Can you work these out from the model? Positions are in its coordinate system, mm. Face numbers are marked on the shaded views. A direction names the side the tool comes from. Round coordinates to 2 decimals unless told otherwise and drop trailing zeros. Order: outer loops, then holes, each group sorted by start corner. A loop starts at its lowest first (then second) coordinate and runs counter-clockwise, first axis right, second up. Notation, with made-up numbers: (53, 86) -> (89, 86) arc R17 cw to (89, 112) -> close; hole circle Ø11 at (-22, -2). An arc over 180 degrees is marked (long way). Use a Markdown table: item, result. Add a question column.
Q1. For the marked faces 1 and 2, which set-ups out of +Z, -Z, +X, -X, +Y, -Y let a thin tool reach every point of the face, with its end or its side?
Q2. I need wall thicknesses on line 1 along Y through (x, z) = (24.5, 23.5); line 2 along X through (y, z) = (32, 51.5). Which ranges of each line are inside material? Lowest first, please. Write a range as [from, to].
Q3. If we section it at A-A on x = 32.5: List the corners of the cut face in (y, z) for me, plus the area to 3 significant figures.
Q4. If we section it at C-C on x = 18: List the corners of the cut face in (y, z) for me.
Q5. If we section it at D-D on y = 38.1: List the corners of the cut face in (x, z) for me, plus the area to 3 significant figures.
Q6. I'm going to push flat-ended pins straight in: pin 1 Ø8 at (x, z) = (45.28, 47.62) entering from -Y; pin 2 Ø4 at (x, z) = (45.28, 47.62) entering from +Y; pin 3 Ø12 at (x, y) = (30, 64.5) entering from -Z. Where does each tip first touch, or does it pass through?
Q7. We'd pull the mould along Y, two halves only. Please class the marked faces 3, 4 and 5: +Y half, -Y half, draft (parallel to the pull), parting line (faces both ways), or undercut.
Q8. If we section it at B-B on z = 31: List the corners of the cut face in (x, y) for me, plus the area to 3 significant figures.
```python
from build123d import *

# Parameters (mm, degrees)
SKETCH2_W               = 50.8
SKETCH2_H               = 76.2
BOSS_EXTRUDE2_DEPTH     = 57.15
SKETCH3_R               = 38.1
CUT_EXTRUDE1_DEPTH      = 108.95
SHELL1_T                = -6.35
F_1_4_CLEARANCE_HOLE1_D = 6.7564


with BuildPart() as part:
    # Sketch2 → Boss-Extrude2 (new body)
    with BuildSketch(Plane.XY):
        with Locations((25.4, 38.1)):
            Rectangle(SKETCH2_W, SKETCH2_H)
    extrude(amount=BOSS_EXTRUDE2_DEPTH)

    # Sketch3 → Cut-Extrude1 (cut, through all)
    with BuildSketch(Plane(origin=(50.8, 0, 0), x_dir=(0, 0, -1), z_dir=(1, 0, 0))):
        with Locations((0, 38.1)):
            Circle(SKETCH3_R)
    extrude(amount=-CUT_EXTRUDE1_DEPTH, mode=Mode.SUBTRACT)

    # Shell1
    shell1_openings = [part.faces().sort_by_distance(p)[0] for p in [
        (25.4, 38.1, 57.15),
        (25.4, 38.1, 38.1),
        (50.8, 38.1, 42.20881959),
    ]]
    offset(amount=SHELL1_T, openings=shell1_openings, kind=Kind.INTERSECTION)

    # 1/4 Clearance Hole1 (through all)
    with Locations(Plane(origin=(0, 76.2, 0), x_dir=(1, 0, 0), z_dir=(0, 1, 0))):
        with Locations((45.28185, -47.625), (19.88185, -47.625)):
            Hole(F_1_4_CLEARANCE_HOLE1_D / 2)


solid = part.part
```
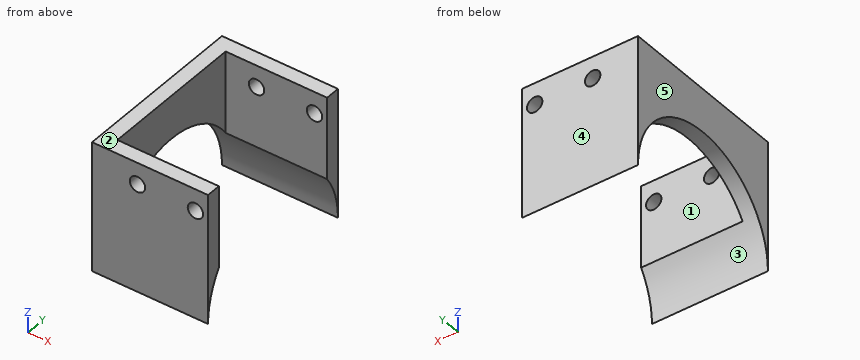
Answer below:
| question | item | result |
|---|---|---|
| 1 | face 1 | +Z, -Z, +X |
| 1 | face 2 | +Z, +X, -X, +Y, -Y |
| 2 | line 1 | [0, 6.35], [69.85, 76.2] |
| 2 | line 2 | [0, 6.35] |
| 3 | outline | (0, 0) arc R38.1 cw to (6.35, 21.06) -> (6.35, 57.15) -> (0, 57.15) -> close; (69.85, 21.06) arc R38.1 cw to (76.2, 0) -> (76.2, 57.15) -> (69.85, 57.15) -> close |
| 3 | area | 544 mm² |
| 4 | outline | (0, 0) arc R38.1 cw to (6.35, 21.06) -> (6.35, 44.82) -> (0, 44.82) -> close; (0, 50.43) -> (6.35, 50.43) -> (6.35, 57.15) -> (0, 57.15) -> close; (69.85, 21.06) arc R38.1 cw to (76.2, 0) -> (76.2, 44.82) -> (69.85, 44.82) -> close; (69.85, 50.43) -> (76.2, 50.43) -> (76.2, 57.15) -> (69.85, 57.15) -> close |
| 5 | outline | (0, 38.1) -> (6.35, 38.1) -> (6.35, 57.15) -> (0, 57.15) -> close |
| 5 | area | 121 mm² |
| 6 | pin 1 | y = 0 |
| 6 | pin 2 | through |
| 6 | pin 3 | z = 20.05 |
| 7 | face 3 | undercut |
| 7 | face 4 | +Y half |
| 7 | face 5 | draft |
| 8 | outline | (0, 0) -> (50.8, 0) -> (50.8, 6.35) -> (6.35, 6.35) -> (6.35, 15.95) -> (0, 15.95) -> close; (0, 60.25) -> (6.35, 60.25) -> (6.35, 69.85) -> (50.8, 69.85) -> (50.8, 76.2) -> (0, 76.2) -> close |
| 8 | area | 767 mm² |
